Verification items for the finished model (mm, model axes). A direction names the side the tool comes from. Coordinates: 2 decimals unless noted, no trailing zeros. Order: outer loops, then holes, each group sorted by start corner. A loop starts at its lowest first (then second) coordinate and runs counter-clockwise, first axis right, second up. Notation, with made-up numbers: M 38.25,58 L 91.25,58 A16 cw 91.25,88 Z; hole C 39.5,-26 d8. An arc over 180 degrees is marked long. Write item = value, one per line.
```python
from build123d import *

# Parameters (mm, degrees)
SKETCH1_W                      = 25
SKETCH1_H                      = 20
BASE_FLANGE1_DEPTH             = 0.7366
EDGE_FLANGE1_STRIP_W           = 4.4196
EDGE_FLANGE1_STRIP_H           = 0.7366
EDGE_FLANGE1_STRIP_CUT_DEPTH   = 20
EDGE_FLANGE1_STRIP_2_W         = 4.4196
EDGE_FLANGE1_STRIP_2_H         = 0.7366
EDGE_FLANGE1_STRIP_CUT_2_DEPTH = 20
EDGE_FLANGE1_DEPTH             = 20
EDGE_FLANGE1_BEND_DEPTH        = 20
F_4_0_4_DIAMETER_HOLE1_D       = 4


# Sheet-metal steps are written as plain solids
with BuildPart() as part:
    # Sketch1 → Base-Flange1 (new body)
    with BuildSketch(Plane(origin=(0, 0, 0), x_dir=(1, 0, 0), z_dir=(0, 1, 0))):
        Rectangle(SKETCH1_W, SKETCH1_H)
    extrude(amount=-BASE_FLANGE1_DEPTH)

    # Edge-Flange1 strip (across the edge) → Edge-Flange1 strip cut (cut)
    with BuildSketch(Plane(origin=(12.5, 0, 10), x_dir=(-1, 0, 0), z_dir=(0, 0, -1))):
        with Locations((-0.7366, -0.3683)):
            Rectangle(EDGE_FLANGE1_STRIP_W, EDGE_FLANGE1_STRIP_H)
    extrude(amount=EDGE_FLANGE1_STRIP_CUT_DEPTH, mode=Mode.SUBTRACT)

    # Edge-Flange1 strip 2 (across the edge) → Edge-Flange1 strip cut 2 (cut)
    with BuildSketch(Plane(origin=(-12.5, 0, -10), x_dir=(1, 0, 0), z_dir=(0, 0, 1))):
        with Locations((-0.7366, -0.3683)):
            Rectangle(EDGE_FLANGE1_STRIP_2_W, EDGE_FLANGE1_STRIP_2_H)
    extrude(amount=EDGE_FLANGE1_STRIP_CUT_2_DEPTH, mode=Mode.SUBTRACT)

    # Edge-Flange1 section (across the edge) → Edge-Flange1 (add)
    with BuildSketch(Plane(origin=(12.5, 0, 10), x_dir=(-1, 0, 0), z_dir=(0, 0, -1))):
        with BuildLine():
            Line((0, 0.7366), (0, 25))
            Line((0, 25), (0.7366, 25))
            Line((0.7366, 25), (0.7366, 0.7366))
            ThreePointArc((0.7366, 0.7366), (0.952345145, 0.215745145), (1.4732, 0))
            Line((1.4732, 0), (1.4732, -0.7366))
            ThreePointArc((1.4732, -0.7366), (0.43149029, -0.30510971), (0, 0.7366))
        make_face()
    extrude(amount=EDGE_FLANGE1_DEPTH)

    # Edge-Flange1 section 2 (across the edge) → Edge-Flange1 bend (add)
    with BuildSketch(Plane(origin=(-12.5, 0, -10), x_dir=(1, 0, 0), z_dir=(0, 0, 1))):
        with BuildLine():
            Line((0, 0.7366), (0, 25))
            Line((0, 25), (0.7366, 25))
            Line((0.7366, 25), (0.7366, 0.7366))
            ThreePointArc((0.7366, 0.7366), (0.952345145, 0.215745145), (1.4732, 0))
            Line((1.4732, 0), (1.4732, -0.7366))
            ThreePointArc((1.4732, -0.7366), (0.43149029, -0.30510971), (0, 0.7366))
        make_face()
    extrude(amount=EDGE_FLANGE1_BEND_DEPTH)

    # Ø4.0 (4) Diameter Hole1 (through all)
    with Locations(Plane(origin=(12.5, 0, 0), x_dir=(0, 0, -1), z_dir=(1, 0, 0))):
        with Locations((0, 17.9834)):
            Hole(F_4_0_4_DIAMETER_HOLE1_D / 2)


solid = part.part
```
Item 1: Sectioned sample at D-D, the plane x = -5.75. Enter the section's corners in (y, z), then the cut area to 3 significant figures.
Report:
outline = M -0.74,-10 L 0,-10 L 0,10 L -0.74,10 Z
area = 14.7 mm^2
Item 2: Release check for a two-part mould opening along Y. For faces 1 (the cylindrical face through (12.127, 19.67, 1.075)), 2 (the flat face through (0, -0.737, 0)), 3 (the flat face through (0.1, -0.2, -10)) record: pulls with the +Y half, pulls with the -Y half, needs draft (parallel to the pull), parting line crosses it, or undercut.
Report:
face_1 = undercut
face_2 = pulls with the -Y half
face_3 = needs draft
Item 3: Sectioned sample at B-B, the plane y = 22.5. Enter the section's corners in (x, z).
Report:
outline = M -12.5,-10 L -11.76,-10 L -11.76,10 L -12.5,10 Z; M 11.76,-10 L 12.5,-10 L 12.5,10 L 11.76,10 Z
Item 4: Sectioned sample at A-A, the plane z = 0. Enter the section's corners in (x, y), then the cut area to 3 significant figures.
Report:
outline = M -12.5,0.74 A1.47 ccw -11.03,-0.74 L 11.03,-0.74 A1.47 ccw 12.5,0.74 L 12.5,15.98 L 11.76,15.98 L 11.76,0.74 A0.74 cw 11.03,0 L -11.03,0 A0.74 cw -11.76,0.74 L -11.76,15.98 L -12.5,15.98 Z; M -12.5,19.98 L -11.76,19.98 L -11.76,25 L -12.5,25 Z; M 11.76,19.98 L 12.5,19.98 L 12.5,25 L 11.76,25 Z
area = 48.7 mm^2
Item 5: Scan lines: L1, parallel to X at y = 13.5, z = 0.5; L2, parallel to Y at x = -12.3, z = 0; L3, parallel to Y at x = -5.75, z = 6.5. Record each from-to range of solid material in increasing order. Write a range as from..to.
Report:
L1 = -12.5..-11.76, 11.76..12.5
L2 = 0..15.98, 19.98..25
L3 = -0.74..0
Item 6: Tool access check on faces 4 (the flat face through (11.763, 13, 0)), 5 (the flat face through (-12.5, 13, 0)). Record the directions out of +Z, -Z, +X, -X, +Y, -Y that give a thin tool (end or side, any length) a straight path to the whole face; none if there is none.
Report:
face_4 = +Z, -Z, +Y
face_5 = +Z, -Z, -X, +Y, -Y
Item 7: Gauge pin test, flat ends, axial feed: pin 1 (10 mm diameter, centred on x = -5, y = 19.5, fed in from +Z); pin 2 (1.5 mm diameter, centred on x = -1.5, z = -6.5, fed in from +Y). Record the tip position at first contact, or that the pin passes through.
Report:
pin_1 = through
pin_2 = 0
Item 8: Sectioned sample at C-C, the plane z = -4.25. Enter the section's corners in (x, y).
Report:
outline = M -12.5,0.74 A1.47 ccw -11.03,-0.74 L 11.03,-0.74 A1.47 ccw 12.5,0.74 L 12.5,25 L 11.76,25 L 11.76,0.74 A0.74 cw 11.03,0 L -11.03,0 A0.74 cw -11.76,0.74 L -11.76,25 L -12.5,25 Z
